Drawing for the job (mm, zero at the part's lowest x, y, z). A direction names the side the tool comes from. Give positions to 0.01 mm unless a question says otherwise; leave off trailing zeros. Order: outer loops, then holes, each group sorted by start corner. A loop starts at its lowest first (then second) coordinate and runs counter-clockwise, first axis right, second up. Notation, with made-up numbers: (1, 18.5) - (53, 18.5) arc R23 cw to (53, 50.5) - close; hole circle Ø10 at (-14, 34). An arc over 180 degrees is marked (long way). One line per item, written item: value.
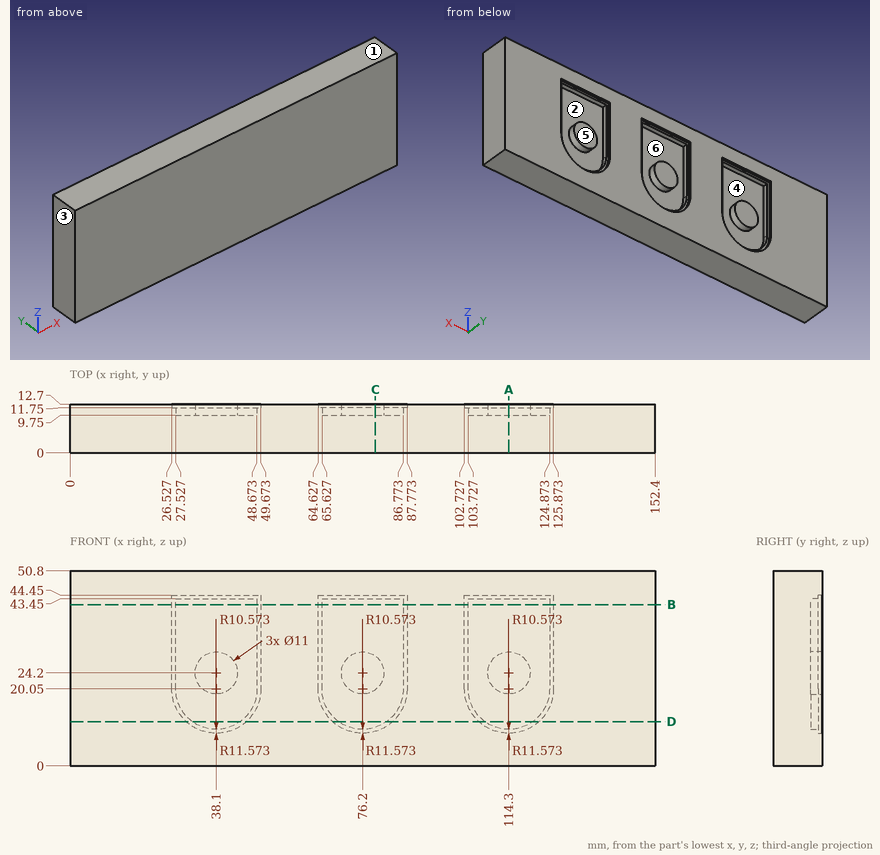
(1) Drill centre lines: line 1 (X direction, y = 11, z = 41.5); line 2 (Z direction, x = 118, y = 10.5); line 3 (Y direction, x = 106.5, z = 12). Where is each one in solid material? Low to high.
Completed:
line 1: 0 to 27.53, 48.67 to 65.63, 86.77 to 103.73, 124.87 to 152.4
line 2: 0 to 10.15, 20.13 to 28.27, 43.45 to 50.8
line 3: 0 to 11.75
(2) Slice it at D-D, the plane z = 11.5. Give the cut face in (x, y), and give its area (3 significant figures).
Completed:
outline: (0, 0) - (152.4, 0) - (152.4, 12.7) - (122.1, 12.7) - (122.1, 11.75) - (120.52, 11.75) - (120.52, 9.75) - (108.08, 9.75) - (108.08, 11.75) - (106.5, 11.75) - (106.5, 12.7) - (84, 12.7) - (84, 11.75) - (82.42, 11.75) - (82.42, 9.75) - (69.98, 9.75) - (69.98, 11.75) - (68.4, 11.75) - (68.4, 12.7) - (45.9, 12.7) - (45.9, 11.75) - (44.32, 11.75) - (44.32, 9.75) - (31.88, 9.75) - (31.88, 11.75) - (30.3, 11.75) - (30.3, 12.7) - (0, 12.7) - close
area: 1,820 mm²
(3) Slice it at C-C, the plane x = 79.5. Give the cut face in (y, z).
Completed:
outline: (0, 0) - (12.7, 0) - (12.7, 8.96) - (11.75, 8.96) - (11.75, 10.01) - (9.75, 10.01) - (9.75, 19.8) - (12.7, 19.8) - (12.7, 28.6) - (9.75, 28.6) - (9.75, 43.45) - (11.75, 43.45) - (11.75, 44.45) - (12.7, 44.45) - (12.7, 50.8) - (0, 50.8) - close
(4) Slice it at A-A, the plane x = 114.3. Give the cut face in (y, z).
Completed:
outline: (0, 0) - (12.7, 0) - (12.7, 8.48) - (11.75, 8.48) - (11.75, 9.48) - (9.75, 9.48) - (9.75, 18.7) - (12.7, 18.7) - (12.7, 29.7) - (9.75, 29.7) - (9.75, 43.45) - (11.75, 43.45) - (11.75, 44.45) - (12.7, 44.45) - (12.7, 50.8) - (0, 50.8) - close
(5) Pin check, flat tip, straight feed: P1, Ø6.5, axis at x = 34, z = 34, coming from the +Y side. Stop position of the tip, or through.
Completed:
P1: y = 9.75
(6) 3-axis set-ups, long thin cutter, end or side, ignore diameter. For the marked faces 1 and 2: which of +Z, -Z, +X, -X, +Y, -Y reach the whole face in a straight line?
Completed:
face 1: +Z, +X, -X, +Y, -Y
face 2: +Y
(7) Slice it at B-B, the plane z = 42. Give the cut face in (x, y).
Completed:
outline: (0, 0) - (152.4, 0) - (152.4, 12.7) - (125.87, 12.7) - (125.87, 11.75) - (124.87, 11.75) - (124.87, 9.75) - (103.73, 9.75) - (103.73, 11.75) - (102.73, 11.75) - (102.73, 12.7) - (87.77, 12.7) - (87.77, 11.75) - (86.77, 11.75) - (86.77, 9.75) - (65.63, 9.75) - (65.63, 11.75) - (64.63, 11.75) - (64.63, 12.7) - (49.67, 12.7) - (49.67, 11.75) - (48.67, 11.75) - (48.67, 9.75) - (27.53, 9.75) - (27.53, 11.75) - (26.53, 11.75) - (26.53, 12.7) - (0, 12.7) - close
(8) Pull direction X, two halves, no side cores. Call the marked faces 3, 4, 5 and 6: +X half, -X half, draft (parallel to the pull), parting line (faces both ways), or undercut.
Completed:
face 3: -X half
face 4: undercut
face 5: draft
face 6: undercut
